Geometry check sheet. Reference: the model listing, model coordinates, mm. Round coordinates to 2 decimals unless told otherwise and drop trailing zeros. Order: outer loops, then holes, each group sorted by start corner. A loop starts at its lowest first (then second) coordinate and runs counter-clockwise, first axis right, second up.
(1) Thickness scan on L1, parallel to Z at x = 49.5, y = -7; L2, parallel to Z at x = 94.5, y = -13.25; L3, parallel to Z at x = 195, y = -13.25. Record the ranges inside material, lowest first.
(2) Cross-section at C-C on x = 184.5. Enter the section's corners in (y, z).
(3) Cross-section at B-B on x = 91.5. Enter the section's corners in (y, z).
(4) Cross-section at A-A on y = -5.25. Enter the section's corners in (x, z), and give its area (3 significant figures).
(5) Gauge pin test, flat ends, axial feed: P1, Ø6.5, axis at x = 67.5, y = -11.5, coming from the -Z side; P2, Ø4.5, axis at x = 120.5, z = -8.5, coming from the -Y side; P3, Ø7.5, axis at x = 193, y = -12.5, coming from the +Z side. Record the tip position at first contact, or that the pin passes through.
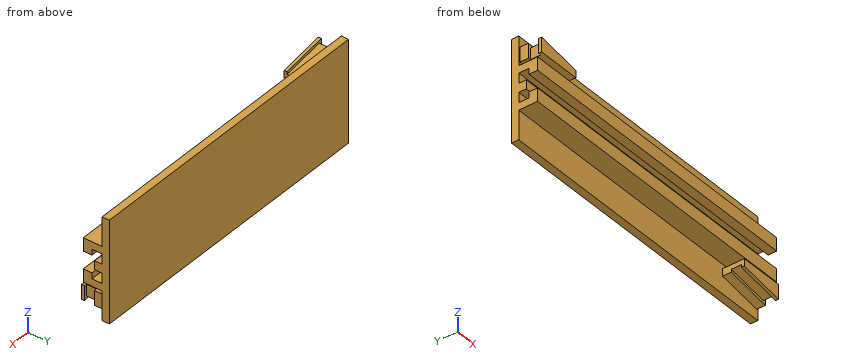
from build123d import *

# Parameters (mm, degrees)
BOSS_EXTRUDE1_DEPTH = 210
BOSS_EXTRUDE2_DEPTH = 15
SKETCH3_W           = 10
SKETCH3_H           = 7
CUT_EXTRUDE1_DEPTH  = 1.8
SKETCH5_W           = 10
SKETCH5_H           = 7
CUT_EXTRUDE2_DEPTH  = 1.8
CUT_EXTRUDE3_DEPTH  = 7
CUT_EXTRUDE4_DEPTH  = 7


with BuildPart() as part:
    # Sketch1 → Boss-Extrude1 (new body)
    with BuildSketch(Plane(origin=(0, 0, 0), x_dir=(0, 0, -1), z_dir=(1, 0, 0))):
        Polygon((-35, -2.5), (-15, -2.5), (-15, -15.5), (-6, -15.5), (-6, -9.5), (-10, -9.5), (-10, -2.5), (-3, -2.5), (-3, -7.710081811), (3, -7.710081811), (3, -2.5), (10, -2.5), (10, -9.5), (6, -9.5), (6, -15.5), (15, -15.5), (15, -2.5), (35, -2.5), (35, 2.5), (-35, 2.5), align=None)
    extrude(amount=BOSS_EXTRUDE1_DEPTH)

    # Sketch2 → Boss-Extrude2 (add)
    with BuildSketch(Plane.XZ.offset(2.5)):
        Polygon((1, 28), (31, 23), (31, 18), (1, 18), align=None)
        Polygon((209, -18), (209, -28), (179, -23), (179, -18), align=None)
    extrude(amount=BOSS_EXTRUDE2_DEPTH)

    # Sketch3 → Cut-Extrude1 (cut)
    with BuildSketch(Plane.ZY.offset(-1)):
        with Locations((23, -12)):
            Rectangle(SKETCH3_W, SKETCH3_H)
    extrude(amount=-CUT_EXTRUDE1_DEPTH, mode=Mode.SUBTRACT)

    # Sketch5 → Cut-Extrude2 (cut)
    with BuildSketch(Plane(origin=(209, 0, 0), x_dir=(0, 0, -1), z_dir=(1, 0, 0))):
        with Locations((23, -12)):
            Rectangle(SKETCH5_W, SKETCH5_H)
    extrude(amount=-CUT_EXTRUDE2_DEPTH, mode=Mode.SUBTRACT)

    # Sketch7 → Cut-Extrude3 (cut)
    with BuildSketch(Plane.XZ.offset(8.5)):
        Polygon((207.2, -27.7), (179, -23), (179, -21.2), (207.2, -25.9), align=None)
    extrude(amount=CUT_EXTRUDE3_DEPTH, mode=Mode.SUBTRACT)

    # Sketch8 → Cut-Extrude4 (cut)
    with BuildSketch(Plane.XZ.offset(8.5)):
        Polygon((2.8, 27.7), (31, 23), (31, 21.2), (2.8, 25.9), align=None)
    extrude(amount=CUT_EXTRUDE4_DEPTH, mode=Mode.SUBTRACT)


solid = part.part
Found:
1. L1: z = -15 to -10, -3 to 3, 10 to 15
1. L2: z = -15 to -6, 6 to 15
1. L3: z = -23.87 to -18, -15 to -6, 6 to 15
2. outline: (-17.5, -23.92) - (-15.5, -23.92) - (-15.5, -22.12) - (-8.5, -22.12) - (-8.5, -23.92) - (-2.5, -23.92) - (-2.5, -35) - (2.5, -35) - (2.5, 35) - (-2.5, 35) - (-2.5, 15) - (-15.5, 15) - (-15.5, 6) - (-9.5, 6) - (-9.5, 10) - (-2.5, 10) - (-2.5, 3) - (-7.71, 3) - (-7.71, -3) - (-2.5, -3) - (-2.5, -10) - (-9.5, -10) - (-9.5, -6) - (-15.5, -6) - (-15.5, -15) - (-2.5, -15) - (-2.5, -18) - (-17.5, -18) - close
3. outline: (-15.5, -15) - (-2.5, -15) - (-2.5, -35) - (2.5, -35) - (2.5, 35) - (-2.5, 35) - (-2.5, 15) - (-15.5, 15) - (-15.5, 6) - (-9.5, 6) - (-9.5, 10) - (-2.5, 10) - (-2.5, 3) - (-7.71, 3) - (-7.71, -3) - (-2.5, -3) - (-2.5, -10) - (-9.5, -10) - (-9.5, -6) - (-15.5, -6) - close
4. outline: (0, -15) - (210, -15) - (210, -10) - (0, -10) - close; (0, -3) - (210, -3) - (210, 3) - (0, 3) - close; (0, 10) - (210, 10) - (210, 15) - (0, 15) - close; (1, 18) - (31, 18) - (31, 23) - (1, 28) - close; (179, -23) - (209, -28) - (209, -18) - (179, -18) - close
4. area: 3,810 mm2
5. P1: stops at z = -15
5. P2: stops at y = -15.5
5. P3: stops at z = 15
